```python
from build123d import *

# Parameters (mm, degrees)
SKETCH_2_W          = 30.48
SKETCH_2_H          = 30.48
EXTRUDE_1_DEPTH     = 5.8
SKETCH_3_R          = 3.1
CUT_EXTRUDE_1_DEPTH = 30.48
CUT_EXTRUDE_2_DEPTH = 2.5
SKETCH_5_R          = 1.6
CUT_EXTRUDE_3_DEPTH = 3.3
FILLET_1_R          = 2.54
CHAMFER_1_SIZE      = 0.6


with BuildPart() as part:
    # 草图2 → 凸台-拉伸1 (new body)
    with BuildSketch(Plane(origin=(0, 0, 0), x_dir=(1, 0, 0), z_dir=(0, 1, 0))):
        Rectangle(SKETCH_2_W, SKETCH_2_H)
    extrude(amount=EXTRUDE_1_DEPTH)

    # 草图3 → 切除-拉伸1 (cut)
    with BuildSketch(Plane.XY.offset(15.24)):
        with Locations((0, 5.9)):
            Circle(SKETCH_3_R)
    extrude(amount=-CUT_EXTRUDE_1_DEPTH, mode=Mode.SUBTRACT)

    # 草图4 → 切除-拉伸2 (cut)
    with BuildSketch(Plane.XZ):
        Polygon((13.567015256, 13.567015256), (10.388253301, 14.418761954), (8.061238046, 12.091746699), (8.912984744, 8.912984744), (12.091746699, 8.061238046), (14.418761954, 10.388253301), align=None)
        Polygon((-13.567015256, 13.567015256), (-14.418761954, 10.388253301), (-12.091746699, 8.061238046), (-8.912984744, 8.912984744), (-8.061238046, 12.091746699), (-10.388253301, 14.418761954), align=None)
        Polygon((13.567015256, -13.567015256), (14.418761954, -10.388253301), (12.091746699, -8.061238046), (8.912984744, -8.912984744), (8.061238046, -12.091746699), (10.388253301, -14.418761954), align=None)
        Polygon((-13.567015256, -13.567015256), (-10.388253301, -14.418761954), (-8.061238046, -12.091746699), (-8.912984744, -8.912984744), (-12.091746699, -8.061238046), (-14.418761954, -10.388253301), align=None)
    extrude(amount=-CUT_EXTRUDE_2_DEPTH, mode=Mode.SUBTRACT)

    # 草图5 → 切除-拉伸3 (cut)
    with BuildSketch(Plane(origin=(0, 2.5, 0), x_dir=(-1, 0, 0), z_dir=(0, -1, 0))):
        with Locations((11.24, -11.24)):
            Circle(SKETCH_5_R)
        with Locations((-11.24, -11.24)):
            Circle(SKETCH_5_R)
        with Locations((-11.24, 11.24)):
            Circle(SKETCH_5_R)
        with Locations((11.24, 11.24)):
            Circle(SKETCH_5_R)
    extrude(amount=-CUT_EXTRUDE_3_DEPTH, mode=Mode.SUBTRACT)

    # 圆角1
    fillet_1_edges = [part.edges().sort_by_distance(p)[0] for p in [
        (15.24, 2.9, 15.24),
        (-15.24, 2.9, 15.24),
        (-15.24, 2.9, -15.24),
        (15.24, 2.9, -15.24),
    ]]
    fillet(fillet_1_edges, radius=FILLET_1_R)

    # 倒角1
    chamfer_1_edges = [part.edges().sort_by_distance(p)[0] for p in [
        (-15.24, 0, 0),
        (15.24, 0, 0),
        (0, 0, 15.24),
        (0, 0, -15.24),
        (14.496051224, 0, -14.496051224),
        (14.496051224, 0, 14.496051224),
        (-14.496051224, 0, 14.496051224),
        (-14.496051224, 0, -14.496051224),
    ]]
    chamfer(chamfer_1_edges, length=CHAMFER_1_SIZE)


solid = part.part
```
Design review of the part built by this model. Coordinates are the model's own, in mm. A direction names the side the tool comes from. Coordinates: 2 decimals unless noted, no trailing zeros. Order: outer loops, then holes, each group sorted by start corner. A loop starts at its lowest first (then second) coordinate and runs counter-clockwise, first axis right, second up. Notation, with made-up numbers: (14, 39.25) -> (20, 39.25) arc R29 ccw to (20, 60.25) -> close; hole circle Ø6 at (-20, 21). An arc over 180 degrees is marked (long way). One line per item, written item: value. Start each with the question number.
Q1. Insertion check: pin 1 Ø3 at (x, z) = (11.24, -11.24) entering from -Y; pin 2 Ø2 at (x, z) = (1, -7.5) entering from +Y; pin 3 Ø1.5 at (x, z) = (0, 1) entering from +Y; pin 4 Ø5 at (x, z) = (11, -11) entering from -Y. Each pin has a flat end and moves straight along its axis. Give the tip position at first contact, or say it passes through.
Q2. Take a section at D-D, the plane x = 11.24. State the section outline as (y, z) points, then the cut area to 3 significant figures.
Q3. Mouldability with a two-part tool opening along X and no side actions: class faces 1 (the flat face through (-10.525, 1.232, 8.481)), 2 (the flat face through (0, 0, 0)), 3 (the flat face through (9.21, 1.23, -13.24)), 4 (the cylindrical face through (-14.516, 3.236, 14.476)) as pulls with the +X half, pulls with the -X half, needs draft (parallel to the pull), parting line crosses it, or undercut.
Q4. Take a section at B-B, the plane y = 3.85. State the section outline as (x, z) points, then the cut area to 3 significant figures.
Q5. Take a section at A-A, the plane y = 2.1. Give the number of separate pieces and of enclosed holes in the cut face, then the cut area to 3 significant figures.
Q6. Tool access review of faces 5 (the cylindrical face through (11.448, 4.127, -12.826)), 6 (the flat face through (12, 1.232, 13.987)): name each direction out of +Z, -Z, +X, -X, +Y, -Y from which nothing blocks a thin tool from reaching the whole face with its end or side.
Q7. Take a section at C-C, the plane z = 11.24. State the section outline as (x, y) points.
Q8. For probe 1 along Z at (x, y) = (-11.24, 4.25); probe 2 along X at (y, z) = (3.4, 11.24); probe 3 along X at (y, z) = (3.85, -11.24), list the stretches that pass through material, from the lowest coordinate up.
Values follow:
1. pin 1: passes through
1. pin 2: stops at y = 3.53
1. pin 3: stops at y = 2.89
1. pin 4: stops at y = 2.5
2. outline: (0, -14.64) -> (0.6, -15.24) -> (5.8, -15.24) -> (5.8, -12.84) -> (2.5, -12.84) -> (2.5, -14.19) -> (0, -14.19) -> close; (0, -8.29) -> (2.5, -8.29) -> (2.5, -9.64) -> (5.8, -9.64) -> (5.8, 9.64) -> (2.5, 9.64) -> (2.5, 8.29) -> (0, 8.29) -> close; (0, 14.19) -> (2.5, 14.19) -> (2.5, 12.84) -> (5.8, 12.84) -> (5.8, 15.24) -> (0.6, 15.24) -> (0, 14.64) -> close
2. area: 126 mm2
3. face 1: undercut
3. face 2: needs draft
3. face 3: undercut
3. face 4: pulls with the -X half
4. outline: (-15.24, -12.7) arc R2.54 ccw to (-12.7, -15.24) -> (-2.33, -15.24) -> (-2.33, 15.24) -> (-12.7, 15.24) arc R2.54 ccw to (-15.24, 12.7) -> close; (2.33, -15.24) -> (12.7, -15.24) arc R2.54 ccw to (15.24, -12.7) -> (15.24, 12.7) arc R2.54 ccw to (12.7, 15.24) -> (2.33, 15.24) -> close; hole circle Ø3.2 at (-11.24, -11.24); hole circle Ø3.2 at (-11.24, 11.24); hole circle Ø3.2 at (11.24, -11.24); hole circle Ø3.2 at (11.24, 11.24)
4. area: 750 mm2
5. separate pieces: 1
5. enclosed holes: 4
5. area: 811 mm2
6. face 5: +Y, -Y
6. face 6: -Y
7. outline: (-15.24, 0.6) -> (-14.64, 0) -> (-14.19, 0) -> (-14.19, 2.5) -> (-12.84, 2.5) -> (-12.84, 5.8) -> (-15.24, 5.8) -> close; (-9.64, 2.5) -> (-8.29, 2.5) -> (-8.29, 0) -> (8.29, 0) -> (8.29, 2.5) -> (9.64, 2.5) -> (9.64, 5.8) -> (3.1, 5.8) arc R3.1 cw to (-3.1, 5.8) -> (-9.64, 5.8) -> close; (12.84, 2.5) -> (14.19, 2.5) -> (14.19, 0) -> (14.64, 0) -> (15.24, 0.6) -> (15.24, 5.8) -> (12.84, 5.8) -> close
8. probe 1: z = -15.24 to -12.84, -9.64 to 9.64, 12.84 to 15.24
8. probe 2: x = -15.24 to -12.84, -9.64 to -1.83, 1.83 to 9.64, 12.84 to 15.24
8. probe 3: x = -15.24 to -12.84, -9.64 to -2.33, 2.33 to 9.64, 12.84 to 15.24
